Autodesk Inventor part; units mm, degrees
ref_plane "YZ Plane" through (0, 0, 0) normal (1, 0, 0) x (0, 1, 0)
ref_plane "XZ Plane" through (0, 0, 0) normal (0, 1, 0) x (-1, 0, 0)
ref_plane "XY Plane" through (0, 0, 0) normal (0, 0, 1) x (1, 0, 0)
sketch "Sketch1" plane through (0, 0, 0) normal (0, 0, 1) x (1, 0, 0)
  line L0 (0, 0) -> (72.4, 0)
  line L1 (72.4, 0) -> (72.4, 71)
  line L2 (72.4, 71) -> (0, 71)
  line L3 (0, 71) -> (0, 0)
  dimension "d0" = 72.4
  dimension "d1" = 71
extrude "Extrusion1" add sketch "Sketch1" along normal blind 10
sketch "Sketch2" plane through (0, 0, 10) normal (0, 0, 1) x (1, 0, 0)
  line L0 (12.4, 71) -> (52.4, 71)
  line L1 (52.4, 71) -> (52.4, 81)
  line L2 (52.4, 81) -> (12.4, 81)
  line L3 (12.4, 81) -> (12.4, 71)
  line L4 (72.4, 0) -> (72.4, 71)
  line L5 (72.4, 71) -> (0, 71)
  circle A0 centre (32.4, 76) radius 2.5
  point P0 (0, 0)
  point P1 (36.2, 71)
  point P2 (52.4, 76)
  point P3 (32.4, 81)
  dimension "d4" = 40
  dimension "d5" = 10
  dimension "d6" = 20
  dimension "d7" = 5
extrude "Extrusion2" add sketch "Sketch2" against normal blind 5
sketch "Sketch3" plane through (0, 0, 10) normal (0, 0, 1) x (1, 0, 0)
  line L0 (72.4, 0) -> (72.4, 71)
  line L1 (72.4, 0) -> (91.4, 0)
  line L2 (91.4, 0) -> (91.4, 62)
  line L3 (91.4, 62) -> (72.4, 62)
  line L4 (72.4, 62) -> (72.4, 0)
  line L5 (72.4, 71) -> (52.4, 71)
  point P0 (0, 0)
  dimension "d10" = 19
  dimension "d11" = 9
extrude "Extrusion3" add sketch "Sketch3" against normal blind 10
sketch "Sketch4" plane through (0, 0, 10) normal (0, 0, 1) x (1, 0, 0)
  line L0 (91.4, 62) -> (72.4, 62)
  circle A0 centre (81.9, 31) radius 2.5
  line L1 (91.4, 0) -> (91.4, 62)
  point P0 (0, 0)
  point P1 (81.9, 62)
  point P2 (91.4, 31)
  dimension "d15" = 5
extrude "Extrusion4" cut sketch "Sketch4" against normal through all
sketch "Sketch5" plane through (0, 0, 10) normal (0, 0, 1) x (1, 0, 0)
  line L0 (0, 0) -> (91.4, 0)
  line L1 (12.4, 0) -> (52.4, 0)
  line L2 (52.4, 0) -> (52.4, 10)
  line L3 (52.4, 10) -> (12.4, 10)
  line L4 (12.4, 10) -> (12.4, 0)
  line L5 (0, 71) -> (0, 0)
  line L6 (0, 55.5) -> (10, 55.5)
  line L7 (10, 55.5) -> (10, 15.5)
  line L8 (10, 15.5) -> (0, 15.5)
  line L9 (0, 15.5) -> (0, 55.5)
  point P0 (52.4, 81)
  point P1 (12.4, 81)
  point P2 (0, 35.5)
  point P3 (0, 35.5)
  dimension "d22" = 10
  dimension "d25" = 10
  dimension "d26" = 40
extrude "Extrusion5" cut sketch "Sketch5" against normal blind 5
sketch "Sketch6" plane through (0, 0, 5) normal (0, 0, 1) x (1, 0, 0)
  line L0 (0, 15.5) -> (0, 55.5)
  line L1 (10, 15.5) -> (0, 15.5)
  line L2 (10, 55.5) -> (10, 15.5)
  line L3 (0, 55.5) -> (10, 55.5)
  line L4 (52.4, 0) -> (12.4, 0)
  line L5 (52.4, 10) -> (52.4, 0)
  line L6 (12.4, 10) -> (52.4, 10)
  line L7 (12.4, 0) -> (12.4, 10)
  circle A0 centre (5, 35.5) radius 2.5
  circle A1 centre (32.4, 5) radius 2.5
  point P0 (0, 0)
  point P1 (0, 35.5)
  point P2 (12.4, 5)
  point P3 (32.4, 10)
  point P4 (5, 55.5)
  dimension "d27" = 5
  dimension "d28" = 5
extrude "Extrusion6" cut sketch "Sketch6" against normal through all contours A0 | A1
properties part number "SP003" material "ABS Plastic"
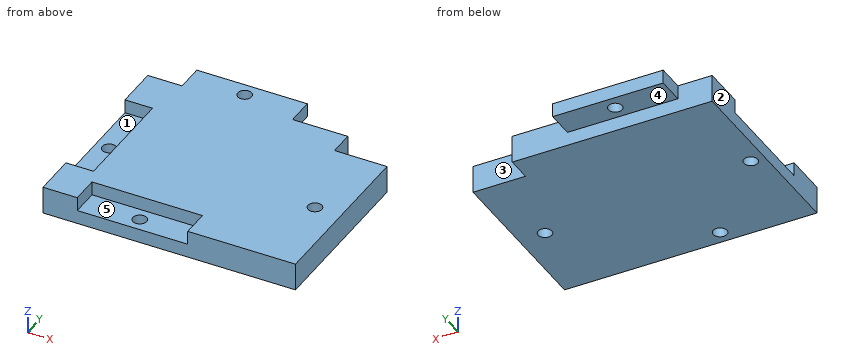
The model under review builds one solid part; all positions refer to its coordinate system, in mm. Face numbers are marked on the shaded views. A direction names the side the tool comes from. Round coordinates to 2 decimals unless told otherwise and drop trailing zeros. Order: outer loops, then holes, each group sorted by start corner. A loop starts at its lowest first (then second) coordinate and runs counter-clockwise, first axis right, second up. Notation, with made-up numbers: (-13.75, 12.25) -> (15.25, 12.25) arc R20 cw to (15.25, 35.25) -> close; hole circle Ø7 at (81, 9). An arc over 180 degrees is marked (long way). Use a Markdown table: item, result.
Q1. We need section D-D on z = 1.25. Write out the cut boundary in (x, y), then the cut area to 3 significant figures.
Values:
| item | result |
|---|---|
| outline | (0, 0) -> (91.4, 0) -> (91.4, 62) -> (72.4, 62) -> (72.4, 71) -> (0, 71) -> close; hole circle Ø5 at (5, 35.5); hole circle Ø5 at (32.4, 5); hole circle Ø5 at (81.9, 31) |
| area | 6,260 mm^2 |
Q2. We need section B-B on x = 81.9. Write out the cut boundary in (y, z), then the cut area to 3 significant figures.
Values:
| item | result |
|---|---|
| outline | (0, 0) -> (28.5, 0) -> (28.5, 10) -> (0, 10) -> close; (33.5, 0) -> (62, 0) -> (62, 10) -> (33.5, 10) -> close |
| area | 570 mm^2 |
Q3. We need section C-C on z = 7. Write out the cut boundary in (x, y).
Values:
| item | result |
|---|---|
| outline | (0, 0) -> (12.4, 0) -> (12.4, 10) -> (52.4, 10) -> (52.4, 0) -> (91.4, 0) -> (91.4, 62) -> (72.4, 62) -> (72.4, 71) -> (52.4, 71) -> (52.4, 81) -> (12.4, 81) -> (12.4, 71) -> (0, 71) -> (0, 55.5) -> (10, 55.5) -> (10, 15.5) -> (0, 15.5) -> close; hole circle Ø5 at (32.4, 76); hole circle Ø5 at (81.9, 31) |
Q4. Tool access review of the marked faces 1, 2, 3, 4 and 5: name each direction out of +Z, -Z, +X, -X, +Y, -Y from which nothing blocks a thin tool from reaching the whole face with its end or side.
Values:
| item | result |
|---|---|
| face 1 | +Z, -X |
| face 2 | +Z, -Z, -X, +Y, -Y |
| face 3 | +Z, -Z, +X, +Y |
| face 4 | -Z, +X, -X, +Y |
| face 5 | +Z, -Y |
Q5. Clearance check with flat-ended pins moving along their axes: P1, Ø6, axis at x = 5, y = 35.5, coming from the +Z side; P2, Ø12, axis at x = 76, y = 71, coming from the -Z side; P3, Ø4.5, axis at x = 81.9, y = 31, coming from the +Z side; P4, Ø1.5, axis at x = 49, z = 6, coming from the -Y side. State where each tip first meets the part, or that it passes through.
Values:
| item | result |
|---|---|
| P1 | stops at z = 5 |
| P2 | stops at z = 0 |
| P3 | passes through |
| P4 | stops at y = 10 |
Q6. We need section A-A on y = 31. Write out the cut boundary in (x, z), then the cut area to 3 significant figures.
Values:
| item | result |
|---|---|
| outline | (0, 0) -> (79.4, 0) -> (79.4, 10) -> (10, 10) -> (10, 5) -> (0, 5) -> close; (84.4, 0) -> (91.4, 0) -> (91.4, 10) -> (84.4, 10) -> close |
| area | 814 mm^2 |
Q7. For line 1 (Y direction, x = 5, z = 1.4); line 2 (Y direction, x = 32.4, z = 1.4); line 3 (Y direction, x = 41, z = 9.5), list the stretches that pass through material, from the lowest coordinate up.
Values:
| item | result |
|---|---|
| line 1 | y = 0 to 33, 38 to 71 |
| line 2 | y = 0 to 2.5, 7.5 to 71 |
| line 3 | y = 10 to 81 |
